Build history of the part. All positions in model axes, mm. A direction names the side the tool comes from. Round coordinates to 2 decimals unless told otherwise and drop trailing zeros. Write each loop counter-clockwise with the first axis right and the second up, starting at its lowest first coordinate (ties: lowest second). Pieces come first, ordered by that corner, then holes. Notation, with made-up numbers: (12, -0.75) - (25, -0.75) arc R7 ccw to (25, 5.25) - close; hole circle Ø5 at (13.5, 56.5). An arc over 180 degrees is marked (long way). Answer as a JSON object with one key per item and string values. Group by question number.
Item 1: Slice it at D-D, the plane y = -0.1. Give the number of separate pieces and of enclosed holes in the cut face, then the cut area to 3 significant figures.
Item 2: Two-plate mould, pull along X, no slides. Class faces 5 (the flat face through (39.5, 0, -5)), 6 (the flat face through (-20, 0, 7)), 7 (the cylindrical face through (-26.93, -0.01, 3.95)): +X half, -X half, draft (parallel to the pull), parting line (faces both ways), or undercut.
Item 3: Probe line 1 (X direction, y = 0, z = -3.5); line 2 (X direction, y = 0.75, z = 6); line 3 (Z direction, x = -1.5, y = 0.5). List the from-to ranges inside material, lowest first. Write a range as from..to.
Item 4: Which spindle directions (+Z, -Z, +X, -X, +Y, -Y) get a long thin tool onto all of the face, cutting with end or side? Do faces 1 (the flat face through (37.8, 0, 9)), 2 (the cylindrical face through (38.25, 0.01, -11.93)), 3 (the flat face through (-3, 0, -7)), 4 (the flat face through (-37.8, 0, 3)). Say none if no direction does.
Item 5: Slice it at A-A, the plane z = 8.5. List the corners of the cut face in (x, y) (3 decimals), then the cut area to 3 significant figures.
Item 6: Slice it at B-B, the plane x = 7.5. List the corners of the cut face in (y, z) (3 decimals).
Item 7: Slice it at C-C, the plane z = -1. List the corners of the cut face in (x, y) (3 decimals).
Item 8: Flat gauge pin, fed straight in: pin 1 (0.8 mm diameter, centred on y = 0.5, z = 3, fed in from -X). Where does the tip first touch, or does it go through?
from build123d import *

# Parameters (mm, degrees)
SKIZZE1_W                       = 5.1
SKIZZE1_H                       = 14
SKIZZE1_W_2                     = 8.35
SKIZZE1_W_3                     = 25
SKIZZE1_H_2                     = 25
AUFSATZ_LINEAR_AUSTRAGEN1_DEPTH = 0.825
VERRUNDUNG1_R                   = 1.5
VERRUNDUNG2_R                   = 0.85


with BuildPart() as part:
    # Skizze1 → Aufsatz-Linear austragen1 (new body, symmetric)
    with BuildSketch(Plane(origin=(0, 0, 0), x_dir=(1, 0, 0), z_dir=(0, 1, 0))):
        Polygon((37.8, 11.5), (37.8, 16.5), (-26.5, 16.5), (-26.5, 14.5), (-26.5, -3.5), (-26.5, -16.5), (37.8, -16.5), (37.8, -0.5), (39.5, -0.5), (39.5, 11.5), align=None)
        with Locations((-19.65, 0)):
            Rectangle(SKIZZE1_W, SKIZZE1_H, mode=Mode.SUBTRACT)
        with Locations((-2.925, 0)):
            Rectangle(SKIZZE1_W_2, SKIZZE1_H, mode=Mode.SUBTRACT)
        with Locations((17.75, 0)):
            Rectangle(SKIZZE1_W_3, SKIZZE1_H_2, mode=Mode.SUBTRACT)
        Polygon((-26.5, -3.5), (-26.5, 14.5), (-37.8, 14.5), (-37.8, 11.5), (-39.5, 11.5), (-39.5, -0.5), (-37.8, -0.5), (-37.8, -3.5), align=None)
    extrude(amount=AUFSATZ_LINEAR_AUSTRAGEN1_DEPTH, both=True)

    # Verrundung1
    verrundung1_edges = [part.edges().sort_by_distance(p)[0] for p in [
        (37.8, 0, -11.5),
        (37.8, 0, 0.5),
        (-26.5, 0, 3.5),
        (-37.8, 0, 0.5),
        (-37.8, 0, -11.5),
        (-26.5, 0, -14.5),
    ]]
    fillet(verrundung1_edges, radius=VERRUNDUNG1_R)

    # Verrundung2
    verrundung2_edges = [part.edges().sort_by_distance(p)[0] for p in [
        (-7.1, 0, -7),
        (-7.1, 0, 7),
        (1.25, 0, 7),
        (1.25, 0, -7),
        (5.25, 0, -12.5),
        (5.25, 0, 12.5),
        (30.25, 0, 12.5),
        (30.25, 0, -12.5),
        (-17.1, 0, 7),
        (-17.1, 0, -7),
        (-22.2, 0, -7),
        (-22.2, 0, 7),
    ]]
    fillet(verrundung2_edges, radius=VERRUNDUNG2_R)


solid = part.part
Geometry says:
{
 "1": {"separate pieces": "1", "enclosed holes": "3", "area": "1,560 mm^2"},
 "2": {"face 5": "+X half", "face 6": "undercut", "face 7": "-X half"},
 "3": {"line 1": "x = -39.5..-22.2, -17.1..-7.1, 1.25..5.25, 30.25..39.5", "line 2": "x = -26.5..-22.2, -17.1..-7.1, 1.25..5.25, 30.25..37.8", "line 3": "z = -16.5..-7, 7..16.5"},
 "4": {"face 1": "+Z, +X, +Y, -Y", "face 2": "-Z, +X, +Y, -Y", "face 3": "+Y, -Y", "face 4": "+Z, -X, +Y, -Y"},
 "5": {"outline": "(-26.5, -0.825) - (5.25, -0.825) - (5.25, 0.825) - (-26.5, 0.825) - close; (30.25, -0.825) - (37.8, -0.825) - (37.8, 0.825) - (30.25, 0.825) - close", "area": "64.8 mm^2"},
 "6": {"outline": "(-0.825, -16.5) - (0.825, -16.5) - (0.825, -12.5) - (-0.825, -12.5) - close; (-0.825, 12.5) - (0.825, 12.5) - (0.825, 16.5) - (-0.825, 16.5) - close"},
 "7": {"outline": "(-39.5, -0.825) - (-22.2, -0.825) - (-22.2, 0.825) - (-39.5, 0.825) - close; (-17.1, -0.825) - (-7.1, -0.825) - (-7.1, 0.825) - (-17.1, 0.825) - close; (1.25, -0.825) - (5.25, -0.825) - (5.25, 0.825) - (1.25, 0.825) - close; (30.25, -0.825) - (39.5, -0.825) - (39.5, 0.825) - (30.25, 0.825) - close"},
 "8": {"pin 1": "stops at x = -37.8"}
}
